Verification items for the finished model (mm, model axes). Coordinates: 2 decimals unless noted, no trailing zeros. Order: outer loops, then holes, each group sorted by start corner. A loop starts at its lowest first (then second) coordinate and runs counter-clockwise, first axis right, second up. Notation, with made-up numbers: M 87,-0.75 L 103,-0.75 A33 cw 103,37.25 Z; hole C 64.25,67.25 d8. An arc over 180 degrees is marked long. Write item = value, one per line.
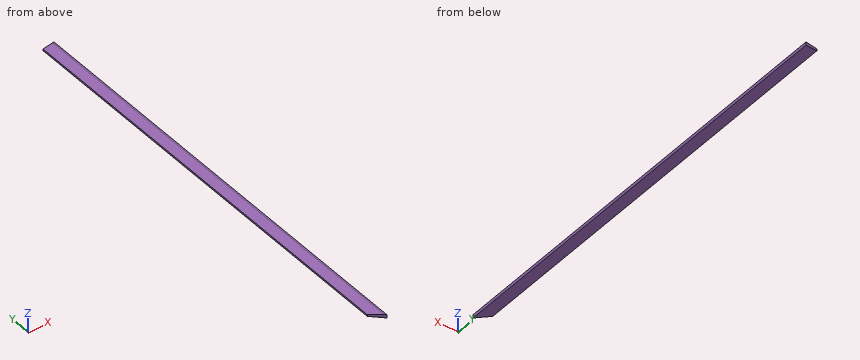
```python
from build123d import *

# Parameters (mm, degrees)
BOSS_EXTRUDE1_DEPTH = 2092.325
CUT_EXTRUDE2_DEPTH  = 2094.081274551


with BuildPart() as part:
    # Sketch1 → Boss-Extrude1 (new body)
    with BuildSketch(Plane(origin=(0, 0, 0), x_dir=(1, 0, 0), z_dir=(0, 1, 0))):
        Polygon((0, 0), (53.975, 0), (53.975, -15.875), (46.355, -15.875), (0, -8.255), align=None)
    extrude(amount=BOSS_EXTRUDE1_DEPTH)

    # Sketch3 → Cut-Extrude2 (cut, through all)
    with BuildSketch(Plane.XY.offset(15.875)):
        Polygon((53.975, 0), (0, 53.975), (0, 0), align=None)
    extrude(amount=-CUT_EXTRUDE2_DEPTH, mode=Mode.SUBTRACT)


solid = part.part
```
Item 1: Sectioned sample at A-A, the plane y = 1808.5. Enter the section's corners in (x, z) (3 decimals).
Report:
outline = M 0,0 L 53.975,0 L 53.975,15.875 L 46.355,15.875 L 0,8.255 Z
Item 2: Sectioned sample at C-C, the plane x = 22. Enter the section's corners in (y, z) (3 decimals).
Report:
outline = M 31.975,0 L 2092.325,0 L 2092.325,11.871 L 31.975,11.871 Z
Item 3: Sectioned sample at B-B, the plane z = 11. Enter the section's corners in (x, y) (3 decimals), then the cut area to 3 significant figures.
Report:
outline = M 16.699,37.276 L 53.975,0 L 53.975,2092.325 L 16.699,2092.325 Z
area = 77,300 mm^2
Item 4: Gauge pin test, flat ends, axial feed: pin 1 (3 mm diameter, centred on x = 8.5, y = 1406, fed in from +Z); pin 2 (4 mm diameter, centred on x = 30.5, y = 1288, fed in from +Z); pin 3 (4 mm diameter, centred on x = 8, z = 13.5, fed in from +Y); pin 4 (2 mm diameter, centred on x = 21.5, y = 1168, fed in from +Z). Record the tip position at first contact, or that the pin passes through.
Report:
pin_1 = 9.9
pin_2 = 13.6
pin_3 = through
pin_4 = 11.95
Item 5: Scan lines: L1, parallel to Y at x = 46.5, z = 11.5 (3 decimals); L2, parallel to Z at x = 46, y = 93; L3, parallel to Z at x = 10, y = 1698. Record each from-to range of solid material in increasing order. Write a range as from..to.
Report:
L1 = 7.475..2092.325
L2 = 0..15.82
L3 = 0..9.9
